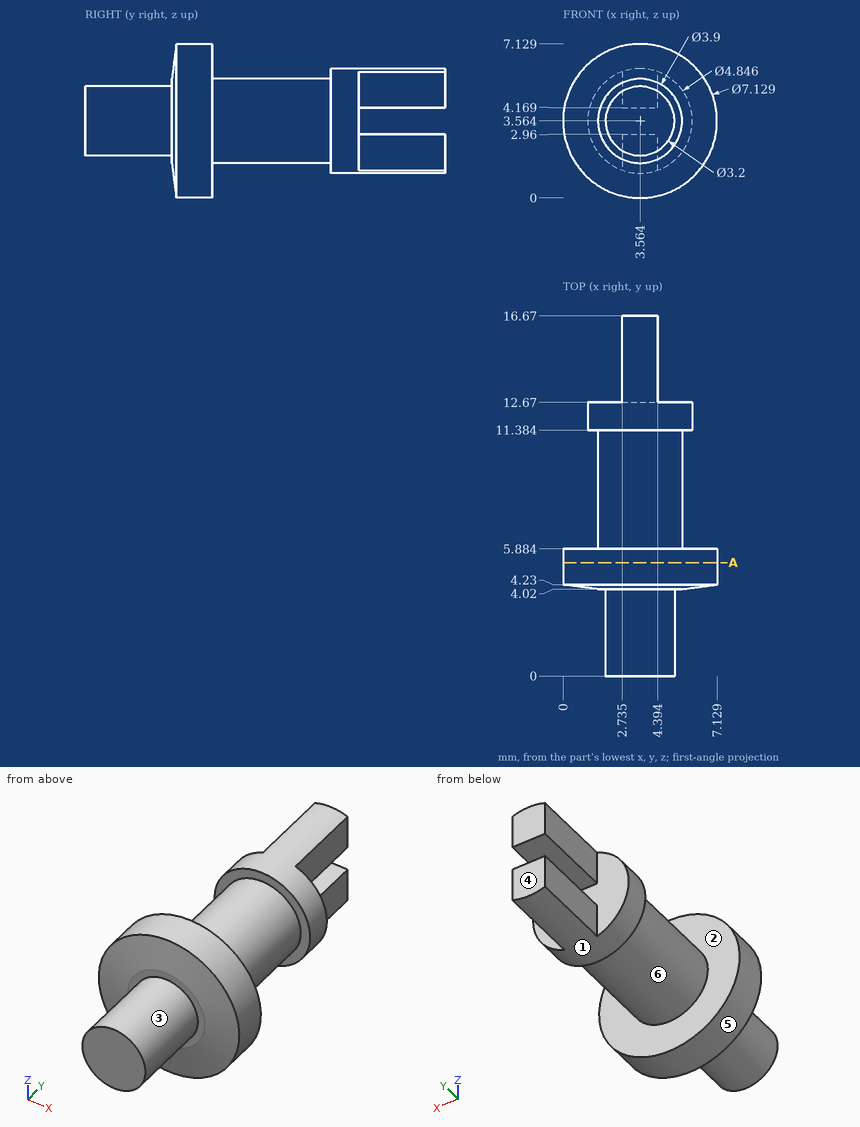
Geometry: see drawing. Coordinates: mm, zero at the bounding-box minimum. A direction names the side the tool comes from. Round coordinates to 2 decimals unless told otherwise and drop trailing zeros. Write each loop counter-clockwise with the first axis right and the second up, starting at its lowest first coordinate (ties: lowest second). Pieces come first, ordered by that corner, then holes.
Item 1: Mould query, pull axis Y, two halves, no side actions, for the marked faces 4, 5 and 6. Classes: +Y half, -Y half, draft (parallel to the pull), parting line (faces both ways), or undercut.
Item 2: Pin query (flat end, axial travel): P1, Ø0.5, axis at y = 14.5, z = 2, coming from the -X side (1 decimal); P2, Ø3, axis at y = 7.5, z = 2.5, coming from the -X side; P3, Ø1.9, axis at x = 3.5, z = 4, coming from the -Y side; P4, Ø1.3, axis at x = 3.5, y = 15.5, coming from the -Z side. Return the tip coordinate at first contact, or that it passes through.
Item 3: Section query A-A (y = 5.25). Return loops of the section in (x, z) (1 decimal), plus the area to 3 significant figures.
Item 4: Material intervals for L1, parallel to X at y = 6.75, z = 3.5 (1 decimal); L2, parallel to X at y = 15.5, z = 5 (1 decimal); L3, parallel to Y at x = 2, z = 1.75 (1 decimal), sorted ascending.
Item 5: Set-up query: the marked faces 1, 2 and 3. Return all of +Z, -Z, +X, -X, +Y, -Y with unobstructed straight access to the full face (end or side cutting, diameter ignored); none if empty.
Completed:
1. face 4: +Y half
1. face 5: draft
1. face 6: undercut
2. P1: stops at x = 2.7
2. P2: stops at x = 1.61
2. P3: stops at y = 0
2. P4: stops at z = 1.14
3. outline: circle Ø7.1 at (3.6, 3.6)
3. area: 39.9 mm2
4. L1: x = 1.6 to 5.5
4. L2: x = 2.7 to 4.4
4. L3: y = 4.1 to 5.9, 11.4 to 12.7
5. face 1: +Y
5. face 2: none
5. face 3: -Y
